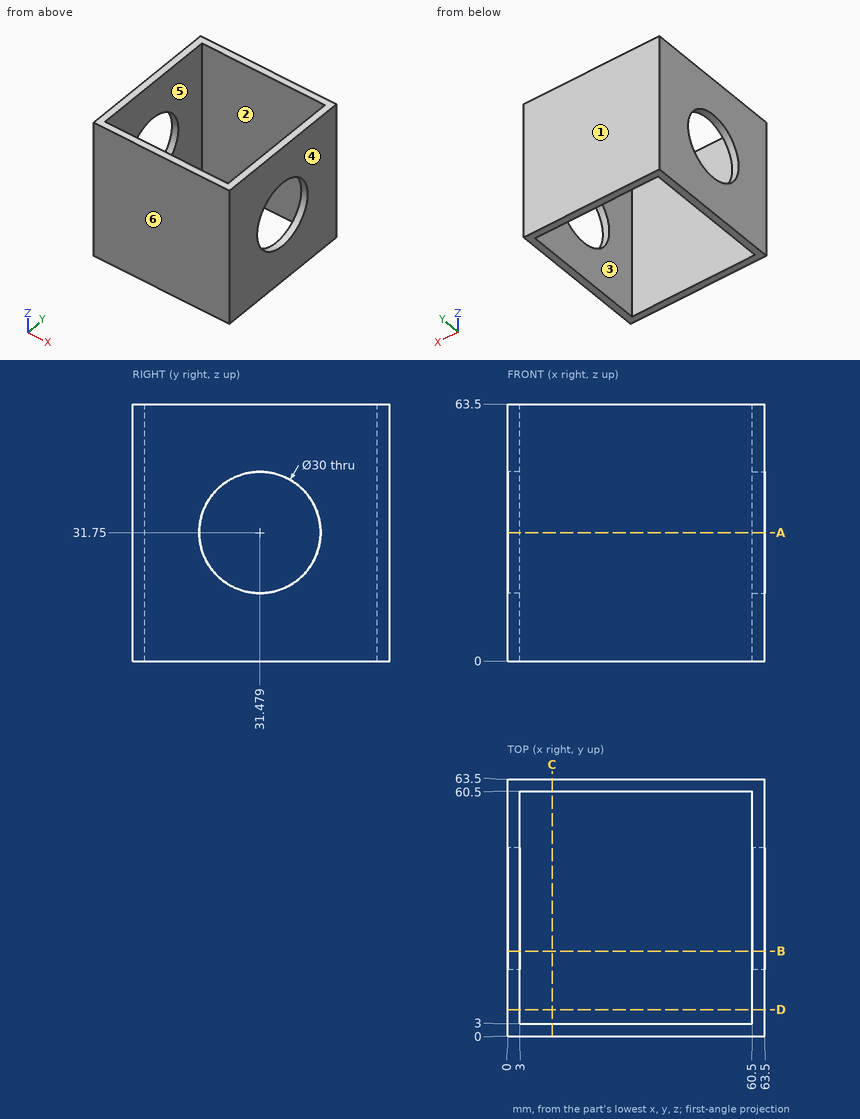
Part print with two shaded views. Sizes in mm from the minimum x, y, z corner. A direction names the side the tool comes from. Coordinates: 2 decimals unless noted, no trailing zeros. Write each loop counter-clockwise with the first axis right and the second up, starting at its lowest first coordinate (ties: lowest second). Pieces come first, ordered by that corner, then holes.
1. Drill centre lines: probe 1 along Y at (x, z) = (18.5, 55); probe 2 along Y at (x, z) = (61, 31). Where is each one in solid material? Low to high.
Answer block:
probe 1: y = 0 to 3, 60.5 to 63.5
probe 2: y = 0 to 16.5, 46.46 to 63.5
2. Pull direction Y, two halves, no side cores. Call the marked faces 3, 4, 5 and 6: released by +Y, released by -Y, zero draft, split by the parting line, or undercut.
Answer block:
face 3: undercut
face 4: zero draft
face 5: undercut
face 6: released by -Y
3. Band-saw the part on A-A, the plane z = 31.75. Give the cut face in (x, y), and give its area (3 significant figures).
Answer block:
outline: (0, 0) - (63.5, 0) - (63.5, 16.48) - (60.5, 16.48) - (60.5, 3) - (3, 3) - (3, 16.48) - (0, 16.48) - close; (0, 46.48) - (3, 46.48) - (3, 60.5) - (60.5, 60.5) - (60.5, 46.48) - (63.5, 46.48) - (63.5, 63.5) - (0, 63.5) - close
area: 546 mm2
4. Band-saw the part on C-C, the plane x = 11. Give the cut face in (y, z), and give its area (3 significant figures).
Answer block:
outline: (0, 0) - (3, 0) - (3, 63.5) - (0, 63.5) - close; (60.5, 0) - (63.5, 0) - (63.5, 63.5) - (60.5, 63.5) - close
area: 381 mm2
5. Drop flat-ended pins along their axis: pin 1 (1 mm diameter, centred on x = 43, z = 17, fed in from -Y); pin 2 (8 mm diameter, centred on x = 10, y = 20, fed in from -Z). Give the stop position or say it passes through.
Answer block:
pin 1: stops at y = 0
pin 2: passes through
6. Band-saw the part on B-B, the plane y = 21. Give the cut face in (x, z), and give its area (3 significant figures).
Answer block:
outline: (0, 0) - (3, 0) - (3, 21.02) - (0, 21.02) - close; (0, 42.48) - (3, 42.48) - (3, 63.5) - (0, 63.5) - close; (60.5, 0) - (63.5, 0) - (63.5, 21.02) - (60.5, 21.02) - close; (60.5, 42.48) - (63.5, 42.48) - (63.5, 63.5) - (60.5, 63.5) - close
area: 252 mm2
7. 3-axis set-ups, long thin cutter, end or side, ignore diameter. For the marked faces 1 and 2: which of +Z, -Z, +X, -X, +Y, -Y reach the whole face in a straight line?
Answer block:
face 1: +Z, -Z, +X, -X, +Y
face 2: +Z, -Z
